Verification items for the finished model (mm, model axes). Face numbers are marked on the shaded views. A direction names the side the tool comes from. Give positions to 0.01 mm unless a question says otherwise; leave off trailing zeros. Write each loop counter-clockwise with the first axis right and the second up, starting at its lowest first coordinate (ties: lowest second). Pieces come first, ordered by that corner, then holes. Notation, with made-up numbers: (62, -7.75) -> (115, -7.75) arc R13 cw to (115, 8.25) -> close; hole circle Ø5 at (62, 30.25). An arc over 180 degrees is marked (long way). Answer as CSV lines item,"result".
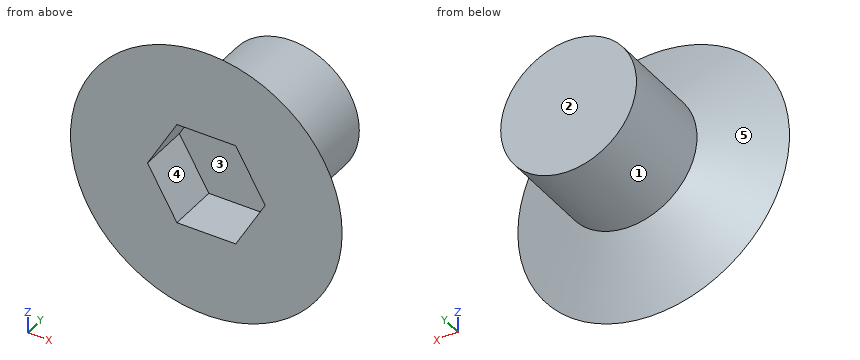
```python
from build123d import *

# Parameters (mm, degrees)
ENL_V_MAT_EXTRU_1_DEPTH = 3


with BuildPart() as part:
    # Esquisse1 → Révolution1 (revolve)
    with BuildSketch(Plane.XY):
        Polygon((0, 0), (8, 0), (4, 2.309401077), (4, 8), (0, 8), align=None)
    revolve(axis=Axis((0, 0, 0), (0, 1, 0)))

    # Esquisse2 → Enlèv. mat.-Extru.1 (cut)
    with BuildSketch(Plane.XZ):
        Polygon((-3.464101615, 0), (-1.732050808, 3), (1.732050808, 3), (3.464101615, 0), (1.732050808, -3), (-1.732050808, -3), align=None)
    extrude(amount=-ENL_V_MAT_EXTRU_1_DEPTH, mode=Mode.SUBTRACT)


solid = part.part
```
1) Section check A-A (x = 0). Record the boundary of the cut face in (y, z), and give its area (3 significant figures).
Reported:
outline,"(0, -8) -> (2.31, -4) -> (8, -4) -> (8, 4) -> (2.31, 4) -> (0, 8) -> (0, 3) -> (3, 3) -> (3, -3) -> (0, -3) -> close"
area,"55.2 mm²"
2) Tool access check on the marked faces 4 and 5. Record the directions out of +Z, -Z, +X, -X, +Y, -Y that give a thin tool (end or side, any length) a straight path to the whole face; none if there is none.
Reported:
face 4,"-Y"
face 5,"+Y"
3) Depth check by flat-ended pin: pin 1 (5 mm diameter, centred on x = 3, z = -1.5, fed in from -Y); pin 2 (4 mm diameter, centred on x = 4, y = 7, fed in from +Z); pin 3 (3 mm diameter, centred on y = 6, z = -1.5, fed in from +X); pin 4 (2 mm diameter, centred on y = 3.5, z = 2, fed in from -X). Enter the tip coordinate at first touch or a pass-through.
Reported:
pin 1,"y = 0"
pin 2,"z = 3.46"
pin 3,"x = 4"
pin 4,"x = -3.87"
4) Draft check along X on the marked faces 1, 2 and 3. Enter one of: +X half, -X half, draft (parallel to the pull), parting line (faces both ways), or undercut.
Reported:
face 1,"parting line"
face 2,"draft"
face 3,"undercut"
5) Scan lines: line 1 along X through (y, z) = (1.5, -2.25); line 2 along Y through (x, z) = (-2.25, -1.25); line 3 along Z through (x, y) = (1, 1). Record each from-to range of solid material in increasing order.
Reported:
line 1,"-4.91 to -2.17, 2.17 to 4.91"
line 2,"3 to 8"
line 3,"-6.19 to -3, 3 to 6.19"
6) Section check B-B (y = 4). Record the boundary of the cut face in (x, z), and give its area (3 significant figures).
Reported:
outline,"circle Ø8 at (0, 0)"
area,"50.3 mm²"
